Design review of the part built by this model. Coordinates are the model's own, in mm. A direction names the side the tool comes from. Coordinates: 2 decimals unless noted, no trailing zeros. Write each loop counter-clockwise with the first axis right and the second up, starting at its lowest first coordinate (ties: lowest second). Pieces come first, ordered by that corner, then holes. Notation, with made-up numbers: (5.25, 13) -> (36.25, 13) arc R18 ccw to (36.25, 31) -> close; hole circle Ø1 at (51.5, -27.75). An arc over 180 degrees is marked (long way). Return JSON: item names as keys, results as strings. Group by question number.
from build123d import *

# Parameters (mm, degrees)
SKETCH_W        = 30
SKETCH_H        = 70
PAD_DEPTH       = 8
PAD001_DEPTH    = 8
SKETCH002_W     = 15
SKETCH002_H     = 43
PAD002_DEPTH    = 6
SKETCH003_R     = 4.1
POCKET_DEPTH    = 70.001
PAD003_DEPTH    = 3.5
CHAMFER_SIZE    = 15
SKETCH005_R     = 3.15
POCKET001_DEPTH = 8.001
SKETCH006_R     = 5.8
POCKET002_DEPTH = 3.6
CHAMFER001_SIZE = 4
CHAMFER002_SIZE = 4
CHAMFER003_SIZE = 3
SKETCH007_W     = 10.5
SKETCH007_H     = 8
SKETCH007_W_2   = 8
SKETCH007_H_2   = 5
SKETCH007_H_3   = 5.5
PAD004_DEPTH    = 2
CHAMFER004_SIZE = 1.9
SKETCH008_W     = 3.080602
SKETCH008_H     = 1
POCKET003_DEPTH = 5.8


with BuildPart() as part:
    # Sketch → Pad (new body)
    with BuildSketch(Plane.XZ):
        with Locations((22.3, 35)):
            Rectangle(SKETCH_W, SKETCH_H)
    extrude(amount=PAD_DEPTH)

    # Sketch001 (on Face6 of Pad) → Pad001 (join)
    with BuildSketch(Plane.XZ.offset(8)):
        Polygon((7.3, 46), (0, 38), (0, 0), (7.3, 0), align=None)
    extrude(amount=-PAD001_DEPTH)

    # Sketch002 (on Face8 of Pad001) → Pad002 (join)
    with BuildSketch(Plane(origin=(0, 0, 0), x_dir=(1, 0, 0), z_dir=(0, 0, -1))):
        with Locations((7.5, 21.5)):
            Rectangle(SKETCH002_W, SKETCH002_H)
    extrude(amount=-PAD002_DEPTH)

    # Sketch003 (on Face10 of Pad002) → Pocket (cut, through all)
    with BuildSketch(Plane(origin=(0, 0, 0), x_dir=(1, 0, 0), z_dir=(0, 0, -1))):
        with Locations((7.85, 34.3)):
            Circle(SKETCH003_R)
    extrude(amount=-POCKET_DEPTH, mode=Mode.SUBTRACT)

    # Sketch004 (on Face8 of Pocket) → Pad003 (join)
    with BuildSketch(Plane(origin=(0, 0, 0), x_dir=(0, 0, -1), z_dir=(-1, 0, 0))):
        Polygon((-6, 8), (-6, 38.4), (-10, 34.4), (-10, 8), align=None)
    extrude(amount=-PAD003_DEPTH)

    # Chamfer
    chamfer_edges = [part.edges().sort_by_distance(p)[0] for p in [
        (15, -8, 3),
    ]]
    chamfer(chamfer_edges, length=CHAMFER_SIZE)

    # Sketch005 (on Face1 of Chamfer) → Pocket001 (cut, through all)
    with BuildSketch(Plane.XZ.offset(8)):
        with Locations((22.3, 35)):
            Circle(SKETCH005_R)
        with Locations((22.3, 60)):
            Circle(SKETCH005_R)
    extrude(amount=-POCKET001_DEPTH, mode=Mode.SUBTRACT)

    # Sketch006 (on Face1 of Pocket001) → Pocket002 (cut)
    with BuildSketch(Plane.XZ.offset(8)):
        with Locations((22.3, 60)):
            Circle(SKETCH006_R)
        with Locations((22.3, 35)):
            Circle(SKETCH006_R)
    extrude(amount=-POCKET002_DEPTH, mode=Mode.SUBTRACT)

    # Chamfer001
    chamfer001_edges = [part.edges().sort_by_distance(p)[0] for p in [
        (37.3, -4, 70),
        (7.3, -4, 70),
        (37.3, -4, 0),
    ]]
    chamfer(chamfer001_edges, length=CHAMFER001_SIZE)

    # Chamfer002
    chamfer002_edges = [part.edges().sort_by_distance(p)[0] for p in [
        (15, -43, 3),
        (0, -43, 3),
    ]]
    chamfer(chamfer002_edges, length=CHAMFER002_SIZE)

    # Chamfer003
    chamfer003_edges = [part.edges().sort_by_distance(p)[0] for p in [
        (0, 0, 19),
    ]]
    chamfer(chamfer003_edges, length=CHAMFER003_SIZE)

    # Sketch007 (on Face5 of Chamfer003) → Pad004 (join)
    with BuildSketch(Plane(origin=(0, 0, 0), x_dir=(1, 0, 0), z_dir=(0, 1, 0))):
        with Locations((12.55, -35)):
            Rectangle(SKETCH007_W, SKETCH007_H)
        with Locations((32.05, -35)):
            Rectangle(SKETCH007_W, SKETCH007_H)
        with Locations((22.3, -53)):
            Rectangle(SKETCH007_W_2, SKETCH007_H_2)
        with Locations((22.3, -67.25)):
            Rectangle(SKETCH007_W_2, SKETCH007_H_3)
    extrude(amount=PAD004_DEPTH)

    # Chamfer004
    chamfer004_edges = [part.edges().sort_by_distance(p)[0] for p in [
        (32.05, 2, 31),
        (12.55, 2, 31),
        (22.3, 2, 50.5),
        (22.3, 2, 64.5),
    ]]
    chamfer(chamfer004_edges, length=CHAMFER004_SIZE)

    # Sketch008 (on Face43 of Chamfer004) → Pocket003 (cut)
    with BuildSketch(Plane(origin=(0, 0, 6), x_dir=(-1, 0, 0), z_dir=(0, 0, 1))):
        with Locations((-13.459699, 34.3)):
            Rectangle(SKETCH008_W, SKETCH008_H)
    extrude(amount=-POCKET003_DEPTH, mode=Mode.SUBTRACT)


solid = part.part
Q1. For faces 1 (the flat face through (2, -21, 10)), 2 (the cylindrical face through (27.832, -6.225, 61.742)), 3 (the flat face through (7.3, 1, 35)), list the 3-axis set-ups (+Z, -Z, +X, -X, +Y, -Y) from which the entire face can be reached by the end or side of a thin tool; tool diameter is ignored.
Q2. The part is to be moulded in two halves that separate along Z. For faces 4 (the flat face through (11, -22, 6)), 5 (the flat face through (35.3, -3.9, 2)), 6 (the flat face through (18.3, 1, 68)), 7 (the flat face through (22, 1, 55.5)), say which applies: +Z half, -Z half, draft (parallel to the pull), parting line (faces both ways), or undercut.
Q3. We need section D-D on y = -20.5. Write out the cut boundary in (x, z).
Q4. For P1, Ø3, axis at x = 11, z = 9.5, coming from the -Y side; P2, Ø8, axis at x = 7, z = 54, coming from the +Y side; P3, Ø15, axis at x = 9, y = -18, coming from the +Z side, all flat-tipped, find the tip position at first contact; note any pin that passes through.
Q5. We need section B-B on y = -6. Write out the cut boundary in (x, z), plus the area to 3 significant figures.
Q6. We need section C-C on x = 32. Write out the cut boundary in (y, z), plus the area to 3 significant figures.
Q7. Wall thickness on L1, parallel to Z at x = 22, y = -5; L2, parallel to Y at x = 7.85, z = 3.4; L3, parallel to Y at x = 32, z = 61: over which ranges is each line inside the solid? List them lowest first.
Q8. We need section A-A on z = 60. Write out the cut boundary in (x, y), plus the area to 3 significant figures.
Findings below:
{
 "1": {"face 1": "+Z, +X, -X, -Y", "face 2": "-Y", "face 3": "+Z, -Z, -X, +Y"},
 "2": {"face 4": "+Z half", "face 5": "-Z half", "face 6": "draft", "face 7": "undercut"},
 "3": {"outline": "(0, 0) -> (17.5, 0) -> (17.5, 6) -> (3.5, 6) -> (3.5, 10) -> (0, 10) -> close"},
 "4": {"P1": "stops at y = -8", "P2": "stops at y = 0", "P3": "stops at z = 10"},
 "5": {"outline": "(0, 0) -> (33.3, 0) -> (37.3, 4) -> (37.3, 66) -> (33.3, 70) -> (11.3, 70) -> (7.3, 66) -> (7.3, 46) -> (0, 38) -> close; hole circle Ø11.6 at (22.3, 35); hole circle Ø11.6 at (22.3, 60)", "area": "2,170 mm^2"},
 "6": {"outline": "(-8, 0) -> (0, 0) -> (0, 31) -> (0.1, 31) -> (2, 32.9) -> (2, 39) -> (0, 39) -> (0, 70) -> (-8, 70) -> close", "area": "574 mm^2"},
 "7": {"L1": "z = 0 to 29.21, 40.79 to 54.21, 65.79 to 70", "L2": "y = -43 to -38.4, -30.2 to 0", "L3": "y = -8 to 0"},
 "8": {"outline": "(7.3, -8) -> (16.5, -8) -> (16.5, -4.4) -> (19.15, -4.4) -> (19.15, 0) -> (7.3, 0) -> close; (25.45, -4.4) -> (28.1, -4.4) -> (28.1, -8) -> (37.3, -8) -> (37.3, 0) -> (25.45, 0) -> close", "area": "171 mm^2"}
}
